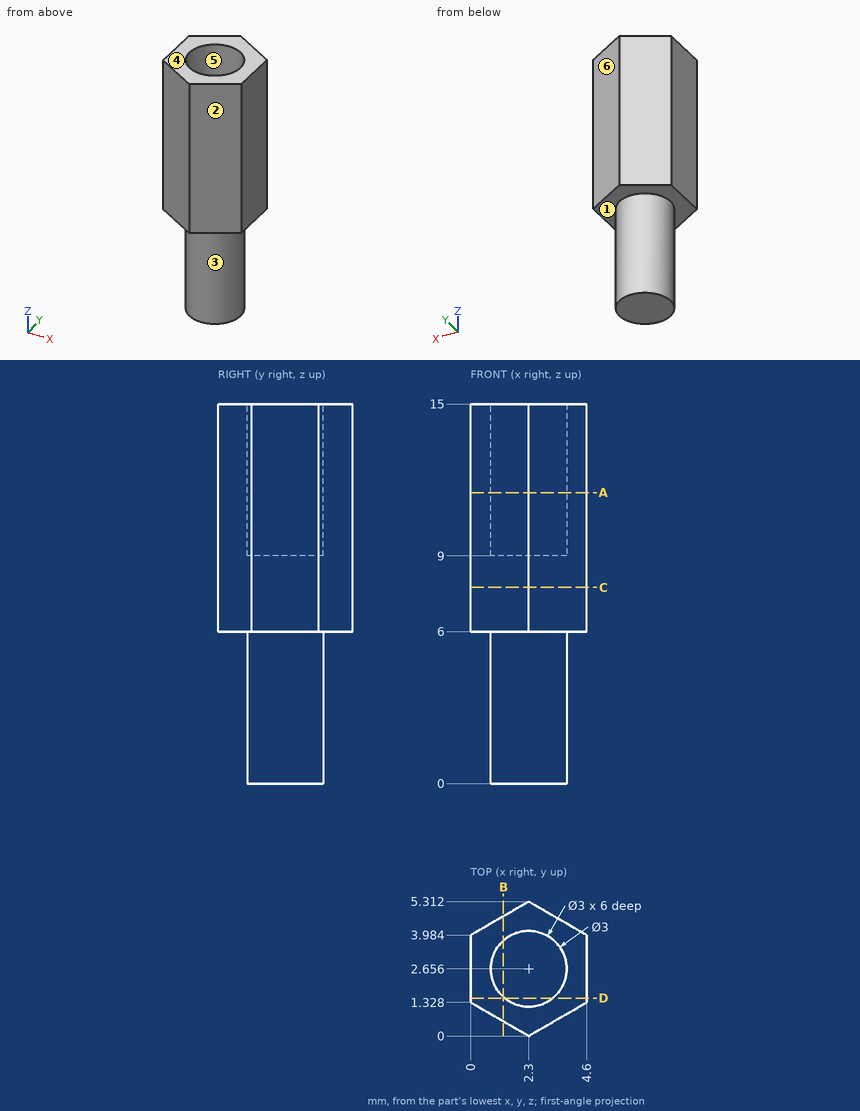
Verification items for this drawing (mm, ordinates from the low corner). A direction names the side the tool comes from. Give positions to 0.01 mm unless a question says otherwise; leave off trailing zeros. Loops run counter-clockwise (first coordinate to the right, second up) from the corner with the lowest first, then second, coordinate; pieces in that order, holes last. Notation, with made-up numbers: M 35.25,-21.5 L 79.25,-21.5 A23 cw 79.25,-11.5 Z; hole C 36.5,-27.5 d8. An arc over 180 degrees is marked long. Write item = value, one per line.
(1) Material ranges on line 1 (Z direction, x = 2.1, y = 2.35); line 2 (Z direction, x = 2.15, y = 0.7); line 3 (X direction, y = 1.4, z = 14.25), recorded low to high. Write a range as [from, to].
Answer below:
line_1 = [0, 9]
line_2 = [6, 15]
line_3 = [0, 1.48], [3.12, 4.6]
(2) Tool access check on the marked faces 1 and 2. Record the directions out of +Z, -Z, +X, -X, +Y, -Y that give a thin tool (end or side, any length) a straight path to the whole face; none if there is none.
Answer below:
face_1 = -Z
face_2 = +Z, -Z, +X, -Y
(3) Sectioned sample at A-A, the plane z = 11.5. Record the cut outline in (x, y) (1 decimal).
Answer below:
outline = M 0,1.3 L 2.3,0 L 4.6,1.3 L 4.6,4 L 2.3,5.3 L 0,4 Z; hole C 2.3,2.7 d3
(4) Release check for a two-part mould opening along X. For the marked faces 3, 4, 5 and 6 record: released by +X, released by -X, zero draft, split by the parting line, or undercut.
Answer below:
face_3 = split by the parting line
face_4 = zero draft
face_5 = undercut
face_6 = released by +X
(5) Sectioned sample at C-C, the plane z = 7.75. Record the cut outline in (x, y).
Answer below:
outline = M 0,1.33 L 2.3,0 L 4.6,1.33 L 4.6,3.98 L 2.3,5.31 L 0,3.98 Z
(6) Sectioned sample at D-D, the plane y = 1.5. Record the cut outline in (x, z).
Answer below:
outline = M 0,6 L 1.34,6 L 1.34,0 L 3.26,0 L 3.26,6 L 4.6,6 L 4.6,15 L 3.26,15 L 3.26,9 L 1.34,9 L 1.34,15 L 0,15 Z
(7) Sectioned sample at B-B, the plane x = 1.3. Record the cut outline in (y, z) (1 decimal).
Answer below:
outline = M 0.6,6 L 1.5,6 L 1.5,0 L 3.8,0 L 3.8,6 L 4.7,6 L 4.7,15 L 3.8,15 L 3.8,9 L 1.5,9 L 1.5,15 L 0.6,15 Z
(8) Gauge pin test, flat end, axial feed: pin 1 Ø1.5 at (x, z) = (3.5, 4.5) entering from +Y. Record the tip position at first contact, or that the pin passes through.
Answer below:
pin_1 = 4.09
